from build123d import *

# Parameters (mm, degrees)
SKETCH_R      = 2.25
SKETCH_R_2    = 57
PAD_DEPTH     = 2
PAD006_DEPTH  = 8
SKETCH014_R   = 4
SKETCH014_R_2 = 2.25
PAD009_DEPTH  = 6
CHAMFER_SIZE  = 0.4


with BuildPart() as part:
    # Sketch → Pad (new body)
    with BuildSketch(Plane.XY):
        with BuildLine():
            Line((-61.9, 38.1), (-61.9, -38.1))
            ThreePointArc((-61.9, -38.1), (-54.929141, -54.929141), (-38.1, -61.9))
            Line((-38.1, -61.9), (38.1, -61.9))
            ThreePointArc((38.1, -61.9), (54.929141, -54.929141), (61.9, -38.1))
            Line((61.9, -38.1), (61.9, 38.1))
            ThreePointArc((61.9, 38.1), (54.929141, 54.929141), (38.1, 61.9))
            Line((38.1, 61.9), (-38.1, 61.9))
            ThreePointArc((-38.1, 61.9), (-54.929141, 54.929141), (-61.9, 38.1))
        make_face()
        with Locations((47.376154, 47.376154)):
            Circle(SKETCH_R, mode=Mode.SUBTRACT)
        Circle(SKETCH_R_2, mode=Mode.SUBTRACT)
    extrude(amount=PAD_DEPTH)

    # Sketch008 → Pad006 (join)
    with BuildSketch(Plane.XY):
        with BuildLine():
            Line((-61.5, 38.1), (-61.5, -38.1))
            ThreePointArc((-61.5, -38.1), (-54.646299, -54.646299), (-38.1, -61.5))
            Line((-38.1, -61.5), (38.1, -61.5))
            ThreePointArc((38.1, -61.5), (54.646299, -54.646299), (61.5, -38.1))
            Line((61.5, -38.1), (61.5, 38.1))
            ThreePointArc((61.5, 38.1), (54.646299, 54.646299), (38.1, 61.5))
            Line((38.1, 61.5), (-38.1, 61.5))
            ThreePointArc((-38.1, 61.5), (-54.646299, 54.646299), (-61.5, 38.1))
        make_face()
        with BuildLine():
            Line((-59.9, 38.1), (-59.9, -38.1))
            ThreePointArc((-59.9, -38.1), (-53.514928, -53.514928), (-38.1, -59.9))
            Line((-38.1, -59.9), (38.1, -59.9))
            ThreePointArc((38.1, -59.9), (53.514928, -53.514928), (59.9, -38.1))
            Line((59.9, -38.1), (59.9, 38.1))
            ThreePointArc((59.9, 38.1), (53.514928, 53.514928), (38.1, 59.9))
            Line((38.1, 59.9), (-38.1, 59.9))
            ThreePointArc((-38.1, 59.9), (-53.514928, 53.514928), (-59.9, 38.1))
        make_face(mode=Mode.SUBTRACT)
    extrude(amount=PAD006_DEPTH)

    # Sketch014 (on Face27 of Pad006) → Pad009 (join)
    with BuildSketch(Plane.XY.offset(2)):
        with Locations((47.376154, 47.376154)):
            Circle(SKETCH014_R)
        with Locations((47.376154, 47.376154)):
            Circle(SKETCH014_R_2, mode=Mode.SUBTRACT)
    extrude(amount=PAD009_DEPTH)

    # Chamfer
    chamfer_edges = [part.edges().sort_by_distance(p)[0] for p in [
        (-57, 0, 2),
        (45.126154, 47.376154, 8),
        (0, 61.5, 8),
        (-61.9, 0, 0),
        (-54.929141, 54.929141, 0),
        (0, 61.9, 0),
        (54.929141, 54.929141, 0),
        (61.9, 0, 0),
        (54.929141, -54.929141, 0),
        (0, -61.9, 0),
        (-54.929141, -54.929141, 0),
        (-57, 0, 0),
        (45.126154, 47.376154, 0),
    ]]
    chamfer(chamfer_edges, length=CHAMFER_SIZE)


solid = part.part
Can you work these out from the model? Positions are in its coordinate system, mm. A direction names the side the tool comes from. Coordinates: 2 decimals unless noted, no trailing zeros. Write each loop counter-clockwise with the first axis right and the second up, starting at its lowest first coordinate (ties: lowest second). Pieces come first, ordered by that corner, then holes. Notation, with made-up numbers: (43.25, 2) -> (72.25, 2) arc R7 cw to (72.25, 10) -> close; hole circle Ø3 at (62, 80.5). An arc over 180 degrees is marked (long way). Write each question's results on one line, items separated by ' | '. Start each with the question number.
Item 1: Please list where these lines run through material, in increasing order: probe 1 along Y at (x, z) = (0, 0.7); probe 2 along Y at (x, z) = (13.5, 4.25).
Item 2: If we section it at A-A, the plane y = 0: Write out the boundary of the cut face in (x, z), and give its area (3 significant figures).
Item 3: On a 3-axis mill with a long thin cutter (end or side, diameter ignored), from which of +Z, -Z, +X, -X, +Y, -Y can I reach the whole of each face in a straight line? I mean faces 4 (the cylindrical face through (54.83, 54.46, 4.76)), 5 (the flat face through (-19, 55, 0)), 6 (the flat face through (0, 58, 2)), 7 (the flat face through (-1, -61.5, 5)). Say none if no direction works.
Item 4: If we section it at B-B, the plane z = 5: Write out the boundary of the cut face in (x, y), and give its area (3 significant figures).
Item 5: Thinking about a two-plate mould opening in Y: for faces 1 (the cylindrical face through (53.345, -53.683, 4.958)), 2 (the cylindrical face through (-54.46, 54.83, 4.76)), 3 (the cylindrical face through (54.743, -55.113, 1.189)), which applies, released by +Y, released by -Y, zero draft, split by the parting line, or undercut?
Item 6: I'm going to push flat-ended pins straight in: P1, Ø1.8, axis at x = 16.5, z = 6, coming from the -Y side; P2, Ø1.7, axis at y = -19, z = 6, coming from the -X side; P3, Ø5, axis at x = 47.38, y = 47.38, coming from the -Z side. Where does each tip first touch, or does it pass through?
Answer block:
1) probe 1: -61.9 to -57, 57 to 61.9 | probe 2: -61.5 to -59.9, 59.9 to 61.5
2) outline: (-61.9, 0.4) -> (-61.5, 0) -> (-57.4, 0) -> (-57, 0.4) -> (-57, 1.6) -> (-57.4, 2) -> (-59.9, 2) -> (-59.9, 8) -> (-61.1, 8) -> (-61.5, 7.6) -> (-61.5, 2) -> (-61.9, 2) -> close; (57, 0.4) -> (57.4, 0) -> (61.5, 0) -> (61.9, 0.4) -> (61.9, 2) -> (61.5, 2) -> (61.5, 7.6) -> (61.1, 8) -> (59.9, 8) -> (59.9, 2) -> (57.4, 2) -> (57, 1.6) -> close | area: 38.2 mm²
3) face 4: +Z, +X, +Y | face 5: -Z, +X, -X, +Y, -Y | face 6: +Z | face 7: +Z, +X, -X, -Y
4) outline: (-61.5, -38.1) arc R23.4 ccw to (-38.1, -61.5) -> (38.1, -61.5) arc R23.4 ccw to (61.5, -38.1) -> (61.5, 38.1) arc R23.4 ccw to (38.1, 61.5) -> (-38.1, 61.5) arc R23.4 ccw to (-61.5, 38.1) -> close; circle Ø8 at (47.38, 47.38); hole (-59.9, -38.1) arc R21.8 ccw to (-38.1, -59.9) -> (38.1, -59.9) arc R21.8 ccw to (59.9, -38.1) -> (59.9, 38.1) arc R21.8 ccw to (38.1, 59.9) -> (-38.1, 59.9) arc R21.8 ccw to (-59.9, 38.1) -> close; hole circle Ø4.5 at (47.38, 47.38) | area: 749 mm²
5) face 1: undercut | face 2: released by +Y | face 3: released by -Y
6) P1: y = -61.5 | P2: x = -61.5 | P3: z = 0.14
